from build123d import *

# Parameters (mm, degrees)
SKETCH1_R           = 1.5875
BOSS_EXTRUDE1_DEPTH = 4.445
BOSS_EXTRUDE2_START = 10.414
BOSS_EXTRUDE2_DEPTH = 10.414
SKETCH1_6_W         = 15.287332686
SKETCH1_6_H         = 3.169044436
SKETCH1_6_W_2       = 7.88471089
BOSS_EXTRUDE3_DEPTH = 24.13
SKETCH4_W           = 13.196572836
SKETCH4_H           = 3.169044436
BOSS_EXTRUDE4_DEPTH = 35.052
SKETCH5_W           = 19.900905811
SKETCH5_H           = 4.632500987
BOSS_EXTRUDE5_DEPTH = 44.704
SKETCH6_R           = 2.54
CUT_EXTRUDE1_DEPTH  = 89.552863771
SKETCH7_R           = 1.994892348
SKETCH7_R_2         = 1.482380007
SKETCH7_R_3         = 1.560959408
CUT_EXTRUDE2_DEPTH  = 87.581521828


with BuildPart() as part:
    # Sketch1 → Boss-Extrude1 (new body)
    with BuildSketch(Plane.XY):
        with BuildLine():
            ThreePointArc((-4.633020552, 14.359873942), (-4.114966432, 12.822559771), (-4.633020552, 11.2852456))
            Line((-4.633020552, 11.2852456), (-4.633020552, 0.224159771))
            Line((-4.633020552, 0.224159771), (18.539023024, 0.224159771))
            Line((18.539023024, 0.224159771), (18.539023024, 28.590004207))
            Line((18.539023024, 28.590004207), (-4.633020552, 28.590004207))
            Line((-4.633020552, 28.590004207), (-4.633020552, 14.359873942))
        make_face()
        with Locations((14.173033568, 21.687159771)):
            Circle(SKETCH1_R, mode=Mode.SUBTRACT)
        with Locations((14.173033568, 3.957959771)):
            Circle(SKETCH1_R, mode=Mode.SUBTRACT)
    extrude(amount=BOSS_EXTRUDE1_DEPTH)

    # Sketch2 → Boss-Extrude2 (add)
    with BuildSketch(Plane(origin=(0, 0, 0), x_dir=(-1, 0, 0), z_dir=(0, 0, -1)).offset(BOSS_EXTRUDE2_START)):
        with BuildLine():
            Line((-18.539023024, 3.433695859), (-15.671467284, 3.433695859))
            ThreePointArc((-15.671467284, 3.433695859), (-14.173033568, 2.370459771), (-12.674599853, 3.433695859))
            Line((-12.674599853, 3.433695859), (4.633020552, 3.433695859))
            Line((4.633020552, 3.433695859), (4.633020552, 0.224159771))
            Line((4.633020552, 0.224159771), (-18.539023024, 0.224159771))
            Line((-18.539023024, 0.224159771), (-18.539023024, 3.433695859))
        make_face()
    extrude(amount=-BOSS_EXTRUDE2_DEPTH)

    # Sketch1_6 → Boss-Extrude3 (add)
    with BuildSketch(Plane.XY):
        with Locations((10.895356681, 27.005481989)):
            Rectangle(SKETCH1_6_W, SKETCH1_6_H)
        with Locations((-0.690665107, 27.005481989)):
            Rectangle(SKETCH1_6_W_2, SKETCH1_6_H)
    extrude(amount=BOSS_EXTRUDE3_DEPTH)

    # Sketch4 → Boss-Extrude4 (add)
    with BuildSketch(Plane.ZY.offset(4.633020552)):
        with Locations((17.531713582, 27.005481989)):
            Rectangle(SKETCH4_W, SKETCH4_H)
    extrude(amount=BOSS_EXTRUDE4_DEPTH)

    # Sketch5 → Boss-Extrude5 (add)
    with BuildSketch(Plane(origin=(0, 28.590004207, 0), x_dir=(1, 0, 0), z_dir=(0, 1, 0))):
        with Locations((-26.955814506, -21.813749507)):
            Rectangle(SKETCH5_W, SKETCH5_H)
    extrude(amount=BOSS_EXTRUDE5_DEPTH)

    # Sketch6 → Cut-Extrude1 (cut, through all)
    with BuildSketch(Plane(origin=(0, 0, 19.497499013), x_dir=(-1, 0, 0), z_dir=(0, 0, -1))):
        with Locations((25.576990215, 60.125767425)):
            Circle(SKETCH6_R)
    extrude(amount=-CUT_EXTRUDE1_DEPTH, mode=Mode.SUBTRACT)

    # Sketch7 → Cut-Extrude2 (cut, through all)
    with BuildSketch(Plane.XZ.offset(-0.224159771)):
        with Locations(Location((-0.152967162, -2.724793136, 0), (0, 0, 270))):
            Circle(SKETCH7_R)
        with Locations(Location((8.696595836, 2.276499013, 0), (0, 0, 270))):
            Circle(SKETCH7_R_2)
        with Locations(Location((8.696595836, -7.723500987, 0), (0, 0, 270))):
            Circle(SKETCH7_R_3)
    extrude(amount=-CUT_EXTRUDE2_DEPTH, mode=Mode.SUBTRACT)


solid = part.part
Source: CAD feature listing. Evaluate the final solid. Frame: model axes, mm. A direction names the side the tool comes from. Give positions to 0.01 mm unless a question says otherwise; leave off trailing zeros. Write each loop counter-clockwise with the first axis right and the second up, starting at its lowest first coordinate (ties: lowest second). Pieces come first, ordered by that corner, then holes. Notation, with made-up numbers: (58, -7) - (111, -7) arc R17 ccw to (111, -2) - close; hole circle Ø8 at (48, -4). An arc over 180 degrees is marked (long way). Write item = value, one per line. Start each with the question number.
Q1. Cut plane A-A, the plane x = 14. Return loops of the section in (y, z) (3 decimals), then the cut area to 3 significant figures.
Q2. Cut plane D-D, the plane x = 3. Return loops of the section in (y, z) (3 decimals).
Q3. Draft query along Y for faces 4 (the cylindrical face through (13.97, 23.26, 2.19)), 5 (the flat face through (7, 16, 0)), 6 (the flat face through (7, 0.224, -3)), 7 (the flat face through (4, 3.434, -5)). Return one class per face: +Y half, -Y half, draft (parallel to the pull), parting line (faces both ways), or undercut.
Q4. Material intervals for probe 1 along Z at (x, y) = (4.5, 19) (3 decimals); probe 2 along Y at (x, z) = (4, 11); probe 3 along Z at (x, y) = (-27.5, 46), sorted ascending.
Q5. Pin query (flat end, axial travel): pin 1 Ø2.5 at (x, z) = (8.7, 2.28) entering from +Y; pin 2 Ø7 at (x, y) = (11, 8.5) entering from +Z (3 decimals); pin 3 Ø8 at (x, z) = (-3.5, 9.5) entering from +Y; pin 4 Ø1 at (x, z) = (1, 6.5) entering from -Y. Return the tip coordinate at first contact, or that it passes through.
Q6. Reachability of faces 1 (the flat face through (-36.906, 51, 22)), 2 (the flat face through (17, 3.434, -5)), 3 (the flat face through (-4.633, 23, 3)) from +Z, -Z, +X, -X, +Y, -Y: full face, straight path, thin tool, end or side. Return the list, or none.
Q7. Cut plane B-B, the plane y = 9. Return loops of the section in (x, z) (1 decimal), then the cut area to 3 significant figures.
Q8. Cut plane C-C, the plane z = 15. Return loops of the section in (x, y), then the cut area to 3 significant figures.
Computed values:
q1.outline = (0.224, -10.414) - (2.38, -10.414) - (2.38, 4.445) - (0.224, 4.445) - close; (5.536, 0) - (20.109, 0) - (20.109, 4.445) - (5.536, 4.445) - close; (23.265, 0) - (28.59, 0) - (28.59, 24.13) - (25.421, 24.13) - (25.421, 4.445) - (23.265, 4.445) - close
q1.area = 183 mm²
q2.outline = (0.224, -10.414) - (3.434, -10.414) - (3.434, 0) - (28.59, 0) - (28.59, 24.13) - (25.421, 24.13) - (25.421, 4.445) - (0.224, 4.445) - close
q3.face_4 = undercut
q3.face_5 = draft
q3.face_6 = -Y half
q3.face_7 = +Y half
q4.probe_1 = 0 to 4.445
q4.probe_2 = 25.42 to 28.59
q4.probe_3 = 19.5 to 24.13
q5.pin_1 = through
q5.pin_2 = 4.445
q5.pin_3 = 28.59
q5.pin_4 = 25.42
q6.face_1 = +Z, -Z, -X, +Y
q6.face_2 = -Z, +X, -X, +Y
q6.face_3 = -Z, -X, +Y, -Y
q7.outline = (-4.6, 0) - (18.5, 0) - (18.5, 4.4) - (-4.6, 4.4) - close; hole circle Ø3 at (8.7, 2.3)
q7.area = 96.1 mm²
q8.outline = (-39.69, 25.42) - (18.54, 25.42) - (18.54, 28.59) - (-39.69, 28.59) - close
q8.area = 185 mm²
